Autodesk Inventor part; units mm, degrees
ref_plane "YZ Plane" through (0, 0, 0) normal (1, 0, 0) x (0, 1, 0)
ref_plane "XZ Plane" through (0, 0, 0) normal (0, 1, 0) x (-1, 0, 0)
ref_plane "XY Plane" through (0, 0, 0) normal (0, 0, 1) x (1, 0, 0)
sketch "Sketch1" plane through (0, 0, 0) normal (1, 0, 0) x (0, 1, 0)
  circle A0 centre (0, 0) radius 12.9812
extrude "Extrusion1" add sketch "Sketch1" along normal blind 10
sketch "Sketch2" plane through (10, 0, 0) normal (1, 0, 0) x (0, 0, -1)
  point P0 (0, 0)
  point P1 (3.4567, 2.9986)
  point P2 (-5.789, 4.4979)
  point P3 (-3.6233, 7.9963)
  point P4 (4.373, -7.9963)
  point P5 (-5.789, -5.9139)
hole "Hole1" at (10, 2.9986, -3.4567) at (10, 4.4979, 5.789) at (10, 7.9963, 3.6233) at (10, -7.9963, -4.373) at (10, -5.9139, 5.789) direction (-1, 0, 0) diameter 3 end through all
properties part number "madeinlinux"
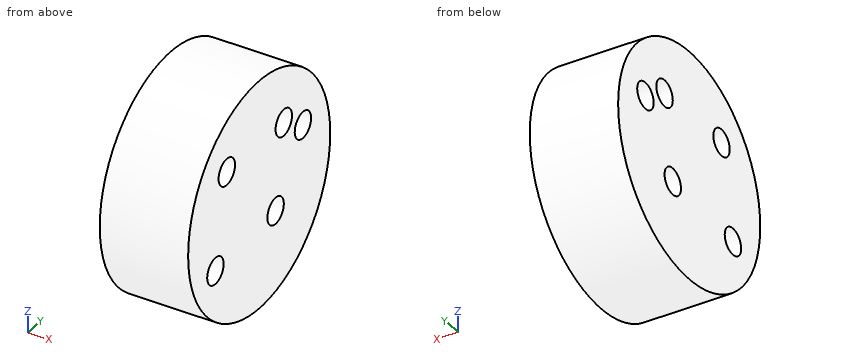
Geometry: final body of the model. Coordinates: model frame, mm. Give positions to 0.01 mm unless a question says otherwise; leave off trailing zeros. Write each loop counter-clockwise with the first axis right and the second up, starting at its lowest first coordinate (ties: lowest second). Pieces come first, ordered by that corner, then holes. Notation, with made-up numbers: (59.25, -38.75) -> (70.25, -38.75) arc R9 cw to (70.25, -34.75) -> close; hole circle Ø1 at (2.25, 81.5). An arc over 180 degrees is marked (long way). Answer in a Markdown table with one row per item.
(1) Pin query (flat end, axial travel): pin 1 (2 mm diameter, centred on x = 6, z = 9, fed in from -Y); pin 2 (1 mm diameter, centred on x = 1.5, y = -4.5, fed in from +Z); pin 3 (2.5 mm diameter, centred on y = 8, z = 3.62, fed in from +X). Return the tip coordinate at first contact, or that it passes through.
Answers below:
| item | result |
|---|---|
| pin 1 | y = -10.22 |
| pin 2 | z = 12.35 |
| pin 3 | through |
(2) Section query D-D on z = -9.25. Return loops of the section in (x, y), then the cut area to 3 significant figures.
Answers below:
| item | result |
|---|---|
| outline | (0, -9.11) -> (10, -9.11) -> (10, 9.11) -> (0, 9.11) -> close |
| area | 182 mm^2 |
(3) Ray query, line 1 along Y through (x, z) = (3.25, -4); line 2 along Y through (x, z) = (1.5, 4.75); line 3 along Z through (x, y) = (7, 7.5). Return the intervals inside material, ascending. Write a range as [from, to].
Answers below:
| item | result |
|---|---|
| line 1 | [-12.35, -9.45], [-6.54, 1.6], [4.4, 12.35] |
| line 2 | [-12.08, -7], [-4.83, 3.42], [5.58, 7.01], [8.99, 12.08] |
| line 3 | [-10.6, 2.21], [5.04, 10.6] |
(4) Section query A-A on z = -3.25. Return loops of the section in (x, y).
Answers below:
| item | result |
|---|---|
| outline | (0, -12.57) -> (10, -12.57) -> (10, -8.99) -> (0, -8.99) -> close; (0, -7) -> (10, -7) -> (10, 1.51) -> (0, 1.51) -> close; (0, 4.48) -> (10, 4.48) -> (10, 12.57) -> (0, 12.57) -> close |
(5) Section query B-B on y = 4. Return loops of the section in (x, z), then the cut area to 3 significant figures.
Answers below:
| item | result |
|---|---|
| outline | (0, -12.35) -> (10, -12.35) -> (10, -4.57) -> (0, -4.57) -> close; (0, -2.34) -> (10, -2.34) -> (10, 4.37) -> (0, 4.37) -> close; (0, 7.2) -> (10, 7.2) -> (10, 12.35) -> (0, 12.35) -> close |
| area | 196 mm^2 |
(6) Section query C-C on x = 8.25. Return loops of the section in (y, z), then the cut area to 3 significant figures.
Answers below:
| item | result |
|---|---|
| outline | circle Ø25.96 at (0, 0); hole circle Ø3 at (-8, -4.37); hole circle Ø3 at (-5.91, 5.79); hole circle Ø3 at (3, -3.46); hole circle Ø3 at (4.5, 5.79); hole circle Ø3 at (8, 3.62) |
| area | 494 mm^2 |
